Can you work these out from the model? Positions are in its coordinate system, mm. Face numbers are marked on the shaded views. A direction names the side the tool comes from. Round coordinates to 2 decimals unless told otherwise and drop trailing zeros. Order: outer loops, then holes, each group sorted by start corner. A loop starts at its lowest first (then second) coordinate and runs counter-clockwise, first axis right, second up.
Q1. If I drill on line 1 (Y direction, x = 9, z = 1.05); line 2 (X direction, y = 32, z = 2.35); line 3 (X direction, y = 29, z = 2), over which ranges is the centre line in solid material (lowest first)?
Q2. For the marked faces 4, 5 and 6, which set-ups out of +Z, -Z, +X, -X, +Y, -Y let a thin tool reach every point of the face, with its end or its side?
Q3. If we section it at A-A (y = 17): Please give me the cut outline in (x, z) (3 decimals).
Q4. If we section it at B-B (y = 28.5): Please give me the cut outline in (x, z) (3 decimals).
Q5. Will this pin go through, and if not, where does the flat tip stop? P1, Ø1, axis at y = 4.5, z = 1, coming from the +X side.
Q6. We'd pull the mould along X, two halves only. Please class the marked faces 1, 2 and 3: pulls with the +X half, pulls with the -X half, needs draft (parallel to the pull), parting line crosses it, or undercut.
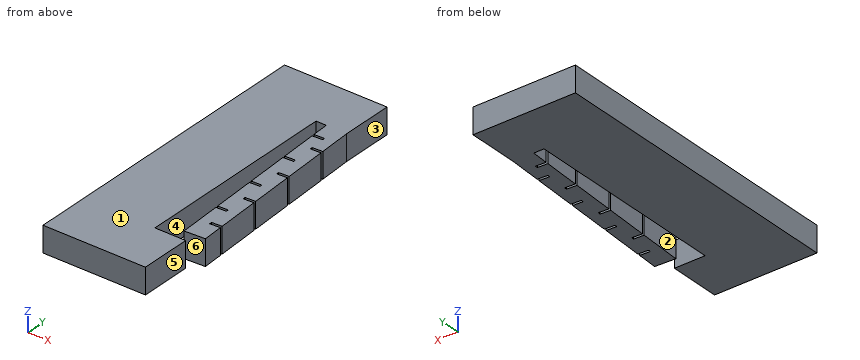
from build123d import *

# Parameters (mm, degrees)
F1_DEPTH = 3.175
F3_DEPTH = 3.176


with BuildPart() as f1:
    # F0 (on Top) → F1 (new body)
    with BuildSketch(Plane.XY):
        Polygon((0, 38.1), (0, 0), (12.7, 0), (12.7, 6.35), (10.16, 6.35), (8.89, 6.35), (8.89, 31.75), (10.16, 31.75), (11.4725997902, 7.6557271994), (14.0088390323, 7.7938955983), (12.7, 31.75), (12.7, 38.1), align=None)
    extrude(amount=F1_DEPTH)

    # F2 (on face) → F3 (cut, through all)
    with BuildSketch(Plane.XY.offset(3.175)):
        Polygon((12.6021534372, 10.2610289821), (13.8702622136, 10.3303119605), (13.8536342988, 10.6346580668), (12.5855255224, 10.5653750884), align=None)
        Polygon((11.1631134086, 13.3367042667), (11.1796827872, 13.0325543411), (12.4478500998, 13.1016411387), (12.431222185, 13.4059872451), align=None)
        Polygon((13.5596651672, 16.0152702235), (13.5430372523, 16.3196163298), (12.2749284759, 16.2503333514), (12.2915563907, 15.9459872451), align=None)
        Polygon((12.1214685819, 19.0909911518), (10.8533966835, 19.0219095522), (10.8699877202, 18.7173620671), (12.1380964967, 18.7866450455), align=None)
        Polygon((13.249065627, 21.7002741302), (13.2324377121, 22.0046202366), (11.9643289357, 21.9353372582), (11.9809568505, 21.6309911518), align=None)
        Polygon((11.8116096197, 24.7796859673), (10.5434899986, 24.7106017678), (10.5600702065, 24.4062530587), (11.8281898276, 24.4753372582), align=None)
        Polygon((11.6701556579, 27.3196859673), (12.9382644344, 27.3889689457), (12.9216365196, 27.693315052), (11.6535277431, 27.6240320736), align=None)
        Polygon((10.2744032886, 29.6499965832), (10.2909834965, 29.3456478741), (11.5591031175, 29.4147320736), (11.5425229097, 29.7190807827), align=None)
        Polygon((12.7241392034, 7.7239081478), (11.4725997902, 7.6557271994), (11.4725997902, 7.3504752393), (12.7407194113, 7.4195594387), align=None)
        Polygon((14.083071413, 6.4351963108), (14.0664434982, 6.7395424171), (12.7983347217, 6.6702594387), (12.8149626365, 6.3659133324), align=None)
    extrude(amount=-F3_DEPTH, mode=Mode.SUBTRACT)


solid = f1.part
Solution:
1. line 1: y = 0 to 6.35, 31.75 to 38.1
1. line 2: x = 0 to 12.7
1. line 3: x = 0 to 8.89, 10.31 to 12.85
2. face 4: +Z, -Z
2. face 5: +Z, -Z, +X, -Y
2. face 6: +Z, -Z, +X
3. outline: (0, 0) - (8.89, 0) - (8.89, 3.175) - (0, 3.175) - close; (10.964, 0) - (13.506, 0) - (13.506, 3.175) - (10.964, 3.175) - close
4. outline: (0, 0) - (8.89, 0) - (8.89, 3.175) - (0, 3.175) - close; (10.337, 0) - (12.878, 0) - (12.878, 3.175) - (10.337, 3.175) - close
5. P1: stops at x = 12.7
6. face 1: needs draft
6. face 2: undercut
6. face 3: pulls with the +X half
